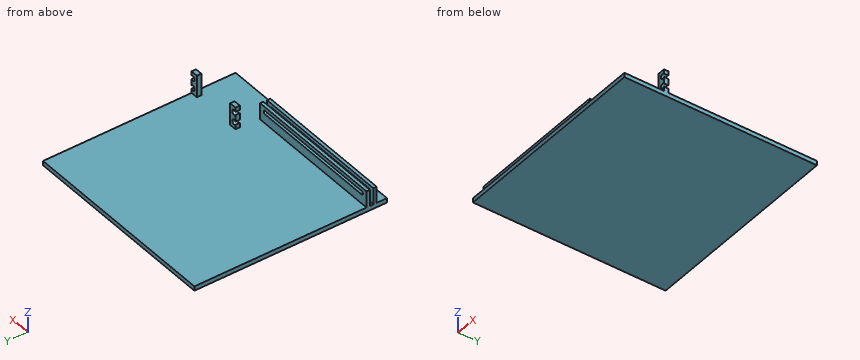
```python
from build123d import *

# Parameters (mm, degrees)
SKETCH_1_W          = 185
SKETCH_1_H          = 175
EXTRUDE_1_DEPTH     = 4
SKETCH_2_W          = 6.45
SKETCH_2_H          = 4
EXTRUDE_2_DEPTH     = 20
CUT_EXTRUDE_1_REACH = 176.157
SKETCH_3_R          = 2.22
SKETCH_4_W          = 130
SKETCH_4_H          = 3
EXTRUDE_3_DEPTH     = 15
CUT_EXTRUDE_2_REACH = 198.044


with BuildPart() as part:
    # 草圖1 → 填料-伸長1 (new body)
    with BuildSketch(Plane.XY):
        with Locations((-9.645986095, 41.11316568)):
            Rectangle(SKETCH_1_W, SKETCH_1_H)
    extrude(amount=EXTRUDE_1_DEPTH)

    # 草圖2 → 填料-伸長2 (add)
    with BuildSketch(Plane.XY.offset(4)):
        with Locations((79.629013905, -8.38683432)):
            Rectangle(SKETCH_2_W, SKETCH_2_H)
        with Locations((32.479013905, -8.38683432)):
            Rectangle(SKETCH_2_W, SKETCH_2_H)
    extrude(amount=EXTRUDE_2_DEPTH)

    # 草圖3 → 除料-伸長1 (cut, up to next)
    with BuildSketch(Plane.XZ.offset(10.38683432), mode=Mode.PRIVATE) as cut_extrude_1_sk1:
        with Locations((81.204013905, 18.5)):
            Circle(SKETCH_3_R)
    cut_extrude_1_tool1 = extrude(cut_extrude_1_sk1.sketch, amount=-CUT_EXTRUDE_1_REACH, mode=Mode.PRIVATE) & part.part
    # 草圖3 → 除料-伸長1 (cut, up to next)
    with BuildSketch(Plane.XZ.offset(10.38683432), mode=Mode.PRIVATE) as cut_extrude_1_sk2:
        with Locations((81.204013905, 9.5)):
            Circle(SKETCH_3_R)
    cut_extrude_1_tool2 = extrude(cut_extrude_1_sk2.sketch, amount=-CUT_EXTRUDE_1_REACH, mode=Mode.PRIVATE) & part.part
    # 草圖3 → 除料-伸長1 (cut, up to next)
    with BuildSketch(Plane.XZ.offset(10.38683432), mode=Mode.PRIVATE) as cut_extrude_1_sk3:
        with Locations((30.904013905, 9.5)):
            Circle(SKETCH_3_R)
    cut_extrude_1_tool3 = extrude(cut_extrude_1_sk3.sketch, amount=-CUT_EXTRUDE_1_REACH, mode=Mode.PRIVATE) & part.part
    # 草圖3 → 除料-伸長1 (cut, up to next)
    with BuildSketch(Plane.XZ.offset(10.38683432), mode=Mode.PRIVATE) as cut_extrude_1_sk4:
        with Locations((30.904013905, 18.5)):
            Circle(SKETCH_3_R)
    cut_extrude_1_tool4 = extrude(cut_extrude_1_sk4.sketch, amount=-CUT_EXTRUDE_1_REACH, mode=Mode.PRIVATE) & part.part
    add(cut_extrude_1_tool1.solids().sort_by_distance((81.204014, -10.386834, 18.5))[0], mode=Mode.SUBTRACT)
    add(cut_extrude_1_tool2.solids().sort_by_distance((81.204014, -10.386834, 9.5))[0], mode=Mode.SUBTRACT)
    add(cut_extrude_1_tool3.solids().sort_by_distance((30.904014, -10.386834, 9.5))[0], mode=Mode.SUBTRACT)
    add(cut_extrude_1_tool4.solids().sort_by_distance((30.904014, -10.386834, 18.5))[0], mode=Mode.SUBTRACT)

    # 草圖4 → 填料-伸長3 (add)
    with BuildSketch(Plane.XY.offset(4)):
        with Locations((-37.145986095, -29.28683432)):
            Rectangle(SKETCH_4_W, SKETCH_4_H)
        with Locations((-37.145986095, -35.48683432)):
            Rectangle(SKETCH_4_W, SKETCH_4_H)
    extrude(amount=EXTRUDE_3_DEPTH)

    # 除料-伸長2: up to this face of the body (flat: up to its plane)
    cut_extrude_2_end = Plane(part.part.faces().sort_by_distance((-37.145986095, -27.78683432, 11.5))[0])
    # 草圖5 → 除料-伸長2 (cut, up to the picked face)
    with BuildSketch(Plane.XZ.offset(36.98683432), mode=Mode.PRIVATE) as cut_extrude_2_sk1:
        with BuildLine():
            Line((-96.145986095, 15.6), (21.854013905, 15.6))
            ThreePointArc((21.854013905, 15.6), (23.454013905, 14), (21.854013905, 12.4))
            Line((21.854013905, 12.4), (-96.145986095, 12.4))
            ThreePointArc((-96.145986095, 12.4), (-97.745986095, 14), (-96.145986095, 15.6))
        make_face()
    cut_extrude_2_tool1 = split(extrude(cut_extrude_2_sk1.sketch, amount=-CUT_EXTRUDE_2_REACH, mode=Mode.PRIVATE), bisect_by=cut_extrude_2_end, keep=Keep.BOTH, mode=Mode.PRIVATE)
    add(cut_extrude_2_tool1.solids().sort_by(Axis((-37.145986, -36.986834, 14), (0, 1, 0)))[0], mode=Mode.SUBTRACT)


solid = part.part
```
Part model, mm, in its own coordinate system. Coordinates: 2 decimals unless noted, no trailing zeros. Order: outer loops, then holes, each group sorted by start corner. A loop starts at its lowest first (then second) coordinate and runs counter-clockwise, first axis right, second up. Notation, with made-up numbers: (45.25, 87.25) -> (87.25, 87.25) arc R24 cw to (87.25, 99.25) -> close; hole circle Ø4 at (70, -18). An arc over 180 degrees is marked (long way). Put each result on its own line as item: value. Start each with the question number.
(1) Band-saw the part on C-C (y = 91). Give the cut face in (x, z).
(2) Band-saw the part on B-B (x = 67.5). Give the cut face in (y, z), then the cut area to 3 significant figures.
(3) Pin check, flat tips, straight feed: pin 1 Ø5 at (x, z) = (30.9, 9.5) entering from +Y; pin 2 Ø1.5 at (x, y) = (-29.5, -36) entering from +Z; pin 3 Ø2.5 at (y, z) = (-36, 8.5) entering from +X; pin 4 Ø2.5 at (x, y) = (-45, -30) entering from -Z. Stop position of each tip, or through.
(4) Band-saw the part on A-A (x = -40.5). Give the cut face in (y, z).
(5) Probe line 1 along Y through (x, z) = (-42, 10.5); line 2 along X through (y, z) = (-8.8, 18.5); line 3 along Z through (x, y) = (-9, 22). List the from-to ranges inside material, lowest first. Write a range as [from, to].
Determined:
1. outline: (-102.15, 0) -> (82.85, 0) -> (82.85, 4) -> (-102.15, 4) -> close
2. outline: (-46.39, 0) -> (128.61, 0) -> (128.61, 4) -> (-46.39, 4) -> close
2. area: 700 mm²
3. pin 1: stops at y = -6.39
3. pin 2: stops at z = 19
3. pin 3: stops at x = 27.85
3. pin 4: stops at z = 0
4. outline: (-46.39, 0) -> (128.61, 0) -> (128.61, 4) -> (-27.79, 4) -> (-27.79, 12.4) -> (-30.79, 12.4) -> (-30.79, 4) -> (-33.99, 4) -> (-33.99, 12.4) -> (-36.99, 12.4) -> (-36.99, 4) -> (-46.39, 4) -> close; (-36.99, 15.6) -> (-33.99, 15.6) -> (-33.99, 19) -> (-36.99, 19) -> close; (-30.79, 15.6) -> (-27.79, 15.6) -> (-27.79, 19) -> (-30.79, 19) -> close
5. line 1: y = [-36.99, -33.99], [-30.79, -27.79]
5. line 2: x = [33.12, 35.7], [76.4, 78.98]
5. line 3: z = [0, 4]
